Verification items for the finished model (mm, model axes). Give positions to 0.01 mm unless a question says otherwise; leave off trailing zeros. Write each loop counter-clockwise with the first axis right and the second up, starting at its lowest first coordinate (ties: lowest second). Pieces come first, ordered by that corner, then holes. Notation, with made-up numbers: (62.5, 55.5) -> (102.5, 55.5) arc R36 cw to (102.5, 93.5) -> close; hole circle Ø4 at (-27, 37.5). An arc over 180 degrees is marked (long way). Use one line per item in the form item = value. Start each with the question number.
(1) Section check A-A, the plane y = 20. Record the cut outline in (x, z) (1 decimal), plus the area to 3 significant figures.
(2) Section check D-D, the plane y = -4. Record the cut outline in (x, z).
(3) Scan lines: L1, parallel to Y at x = -35, z = 0.2; L2, parallel to X at y = -3, z = 4; L3, parallel to X at y = 7, z = 2.7. Record each from-to range of solid material in increasing order.
(4) Section check C-C, the plane x = 13. Record the cut outline in (y, z).
(5) Depth check by flat-ended pin: pin 1 Ø2.5 at (y, z) = (-20.5, 2.5) entering from +X; pin 2 Ø1 at (y, z) = (15, 1.5) entering from -X; pin 3 Ø1 at (y, z) = (-3.5, 1) entering from +X; pin 4 Ø1.5 at (x, y) = (31.5, -7) entering from -Z. Enter the tip coordinate at first touch or a pass-through.
from build123d import *

# Parameters (mm, degrees)
SKETCH2_W           = 85
SKETCH2_H           = 35
SKETCH2_W_2         = 5
SKETCH2_H_2         = 17.45
SKETCH2_W_3         = 9.85
SKETCH2_H_3         = 5
BOSS_EXTRUDE1_DEPTH = 5


with BuildPart() as part:
    # Sketch2 → Boss-Extrude1 (new body)
    with BuildSketch(Plane.XY):
        Rectangle(SKETCH2_W, SKETCH2_H)
        with Locations((-45, -8.775)):
            Rectangle(SKETCH2_W_2, SKETCH2_H_2)
        with Locations((-26.2125, 20)):
            Rectangle(SKETCH2_W_3, SKETCH2_H_3)
        with Locations((0, 20)):
            Rectangle(SKETCH2_W_3, SKETCH2_H_3)
        with Locations((26.2125, 20)):
            Rectangle(SKETCH2_W_3, SKETCH2_H_3)
        with Locations((45, 8.775)):
            Rectangle(SKETCH2_W_2, SKETCH2_H_2)
        with Locations((26.2125, -20)):
            Rectangle(SKETCH2_W_3, SKETCH2_H_3)
        with Locations((0, -20)):
            Rectangle(SKETCH2_W_3, SKETCH2_H_3)
        with Locations((-26.2125, -20)):
            Rectangle(SKETCH2_W_3, SKETCH2_H_3)
    extrude(amount=BOSS_EXTRUDE1_DEPTH)


solid = part.part
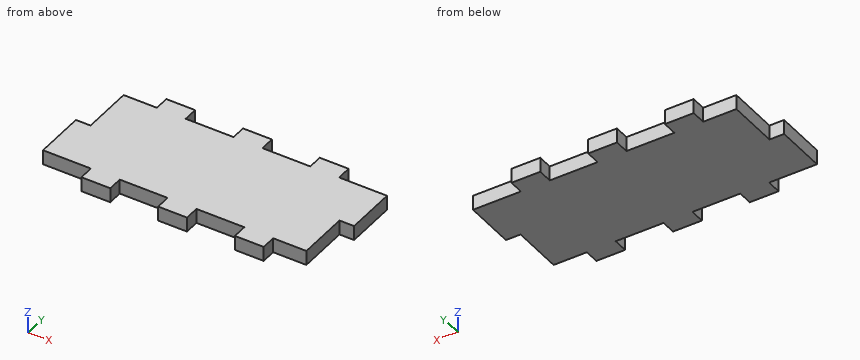
Completed:
q1.outline = (-31.1, 0) -> (-21.3, 0) -> (-21.3, 5) -> (-31.1, 5) -> close; (-4.9, 0) -> (4.9, 0) -> (4.9, 5) -> (-4.9, 5) -> close; (21.3, 0) -> (31.1, 0) -> (31.1, 5) -> (21.3, 5) -> close
q1.area = 148 mm²
q2.outline = (-47.5, 0) -> (42.5, 0) -> (42.5, 5) -> (-47.5, 5) -> close
q3.L1 = -17.5 to 17.5
q3.L2 = -47.5 to 42.5
q3.L3 = -42.5 to 47.5
q4.outline = (-17.5, 0) -> (17.5, 0) -> (17.5, 5) -> (-17.5, 5) -> close
q5.pin_1 = 31.14
q5.pin_2 = -42.5
q5.pin_3 = 42.5
q5.pin_4 = 0
